Input: part model. Units: mm. Frame: model coordinates. Face numbers are marked on the shaded views. A direction names the side the tool comes from. Round coordinates to 2 decimals unless told otherwise and drop trailing zeros. Write each loop counter-clockwise with the first axis right and the second up, starting at its lowest first coordinate (ties: lowest second). Pieces come first, ordered by that corner, then holes. Notation, with made-up numbers: (49, -10) - (65, -10) arc R26 ccw to (65, 7) - close; hole circle Ø9 at (-9.75, 76). An arc over 180 degrees is marked (long way). One line per item, written item: value. Start each with the question number.
```python
from build123d import *

# Parameters (mm, degrees)
SKETCH_1_R           = 7.5
SKETCH_1_R_2         = 4.1
EXTRUDE_1_DEPTH      = 20
EXTRUDE_2_DEPTH      = 6
EXTRUDE_2_DEPTH_BACK = 6
SKETCH_2_W           = 20
SKETCH_2_H           = 20
SKETCH_2_R           = 2
SKETCH_3_W           = 20
SKETCH_3_H           = 3.1
CUT_EXTRUDE_1_DEPTH  = 15


with BuildPart() as part:
    # Sketch 1 → Extrude 1 (new body)
    with BuildSketch(Plane.XY):
        Circle(SKETCH_1_R)
        Circle(SKETCH_1_R_2, mode=Mode.SUBTRACT)
    extrude(amount=EXTRUDE_1_DEPTH)

    # Sketch 2 → Extrude 2 (add, two sides: drawn at the far end of the back side and taken through both)
    with BuildSketch(Plane(origin=(0, 0, 0), x_dir=(1, 0, 0), z_dir=(0, 1, 0)).offset(-EXTRUDE_2_DEPTH_BACK)):
        with Locations((14.1, -10)):
            Rectangle(SKETCH_2_W, SKETCH_2_H)
        with Locations(Location((18, -10, 0), (0, 0, 270))):
            Circle(SKETCH_2_R, mode=Mode.SUBTRACT)
    extrude(amount=EXTRUDE_2_DEPTH + EXTRUDE_2_DEPTH_BACK)

    # Sketch 3 → Cut-Extrude 1 (cut)
    with BuildSketch(Plane(origin=(24.1, 0, 0), x_dir=(0, 0, -1), z_dir=(1, 0, 0))):
        with Locations((-10, -0.077105761)):
            Rectangle(SKETCH_3_W, SKETCH_3_H)
    extrude(amount=-CUT_EXTRUDE_1_DEPTH, mode=Mode.SUBTRACT)


solid = part.part
```
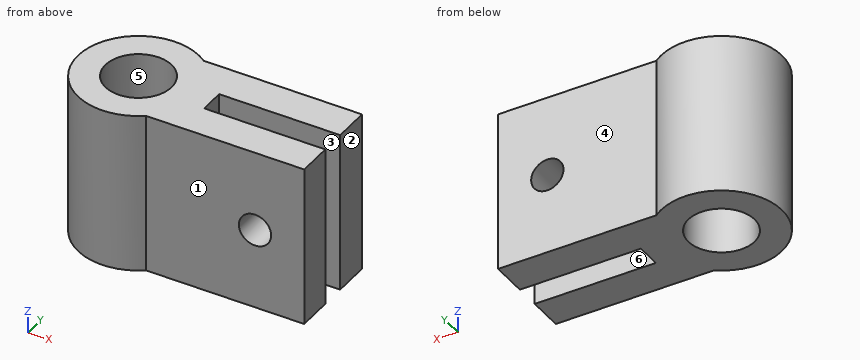
Q1. Pull-direction query (Y, two-part tool) for the marked faces 1, 2 and 3; classes: pulls with the +Y half, pulls with the -Y half, needs draft (parallel to the pull), parting line crosses it, or undercut.
Q2. Cut plane D-D, the plane y = 2.75. Output: boundary loops of the cut face in (x, z), and give its area (3 significant figures).
Q3. Cut plane C-C, the plane x = 18. Output: boundary loops of the cut face in (y, z), and give its area (3 significant figures).
Q4. Access query for the marked faces 4, 5 and 6. Directions: +Z, -Z, +X, -X, +Y, -Y. A direction counts if a zero-diameter tool reaches every point of the face in a straight line with its end or side. Return the directions, or none.
Q5. Cut plane B-B, the plane y = 0. Output: boundary loops of the cut face in (x, z).
Q6. Material intervals for probe 1 along Y at (x, z) = (9.5, 8.5); probe 2 along Z at (x, y) = (18, 2.5); probe 3 along X at (y, z) = (-1, 10.5), sorted ascending. Write a range as from..to.
Q7. Contact query for flat-ended pins moving along their axis: pin 1 Ø1.6 at (y, z) = (0, 13.5) entering from +X; pin 2 Ø3.5 at (x, z) = (18, 10) entering from +Y; pin 3 Ø5 at (x, z) = (18, 10) entering from -Y; pin 4 Ø1.5 at (y, z) = (-6, 6.5) entering from -X. Output: stop coordinate, or through.
Q8. Cut plane A-A, the plane z = 10. Output: boundary loops of the cut face in (x, y), and give its area (3 significant figures).
A:
1. face 1: pulls with the -Y half
1. face 2: needs draft
1. face 3: undercut
2. outline: (-6.98, 0) - (-3.04, 0) - (-3.04, 20) - (-6.98, 20) - close; (3.04, 0) - (24.1, 0) - (24.1, 20) - (3.04, 20) - close; hole circle Ø4 at (18, 10)
2. area: 487 mm²
3. outline: (-6, 0) - (-1.63, 0) - (-1.63, 8) - (-6, 8) - close; (-6, 12) - (-1.63, 12) - (-1.63, 20) - (-6, 20) - close; (1.47, 0) - (6, 0) - (6, 8) - (1.47, 8) - close; (1.47, 12) - (6, 12) - (6, 20) - (1.47, 20) - close
3. area: 142 mm²
4. face 4: +Z, -Z, +X, +Y
4. face 5: +Z, -Z
4. face 6: +Z, -Z, +X
5. outline: (-7.5, 0) - (-4.1, 0) - (-4.1, 20) - (-7.5, 20) - close; (4.1, 0) - (9.1, 0) - (9.1, 20) - (4.1, 20) - close
6. probe 1: y = -6..-1.63, 1.47..6
6. probe 2: z = 0..8, 12..20
6. probe 3: x = -7.43..-3.98, 3.98..9.1
7. pin 1: stops at x = 9.1
7. pin 2: passes through
7. pin 3: stops at y = -6
7. pin 4: stops at x = -5.36
8. outline: (4.5, -6) - (16, -6) - (16, -1.63) - (9.1, -1.63) - (9.1, 1.47) - (16, 1.47) - (16, 6) - (4.5, 6) arc R7.5 ccw (long way) to start; (20, -6) - (24.1, -6) - (24.1, -1.63) - (20, -1.63) - close; (20, 1.47) - (24.1, 1.47) - (24.1, 6) - (20, 6) - close; hole circle Ø8.2 at (0, 0)
8. area: 252 mm²
